from build123d import *

# Parameters (mm, degrees)
SKETCH1_W           = 45
SKETCH1_H           = 250
BOSS_EXTRUDE1_DEPTH = 12
SKETCH2_W           = 5
SKETCH2_H           = 105
CUT_EXTRUDE1_DEPTH  = 12
SKETCH3_R           = 1.75
CUT_EXTRUDE2_DEPTH  = 35
SKETCH5_W           = 25
SKETCH5_H           = 30
SKETCH5_W_2         = 5
BOSS_EXTRUDE2_DEPTH = 12
SKETCH7_R           = 12
SKETCH7_R_2         = 1.25
CUT_EXTRUDE3_DEPTH  = 35
SKETCH8_W           = 18
SKETCH8_H           = 11
CUT_EXTRUDE4_DEPTH  = 12
SKETCH10_R          = 11
CUT_EXTRUDE5_DEPTH  = 7
SKETCH11_W          = 45
SKETCH11_H          = 20
CUT_EXTRUDE6_DEPTH  = 20
FILLET3_R           = 5
SKETCH12_R          = 5
CUT_EXTRUDE7_DEPTH  = 10
SKETCH13_R          = 1.5
CUT_EXTRUDE8_DEPTH  = 12
CUT_EXTRUDE9_DEPTH  = 20
FILLET4_R           = 18
SKETCH15_R          = 5
CUT_EXTRUDE10_DEPTH = 10


with BuildPart() as part:
    # Sketch1 → Boss-Extrude1 (new body)
    with BuildSketch(Plane(origin=(0, 0, 0), x_dir=(1, 0, 0), z_dir=(0, 1, 0))):
        Rectangle(SKETCH1_W, SKETCH1_H)
    extrude(amount=BOSS_EXTRUDE1_DEPTH)

    # Sketch2 → Cut-Extrude1 (cut)
    with BuildSketch(Plane(origin=(0, 12, 0), x_dir=(1, 0, 0), z_dir=(0, 1, 0))):
        with Locations((20, 42.5)):
            Rectangle(SKETCH2_W, SKETCH2_H)
        with Locations((-20, 42.5)):
            Rectangle(SKETCH2_W, SKETCH2_H)
    extrude(amount=-CUT_EXTRUDE1_DEPTH, mode=Mode.SUBTRACT)

    # Sketch3 → Cut-Extrude2 (cut)
    with BuildSketch(Plane(origin=(17.5, 0, 0), x_dir=(0, 0, -1), z_dir=(1, 0, 0))):
        with Locations((15, 6)):
            Circle(SKETCH3_R)
        with Locations((75, 6)):
            Circle(SKETCH3_R)
    extrude(amount=-CUT_EXTRUDE2_DEPTH, mode=Mode.SUBTRACT)

    # Sketch5 → Boss-Extrude2 (add)
    with BuildSketch(Plane(origin=(0, 12, 0), x_dir=(1, 0, 0), z_dir=(0, 1, 0))):
        with Locations((35, 110)):
            Rectangle(SKETCH5_W, SKETCH5_H)
        with Locations((-25, 110)):
            Rectangle(SKETCH5_W_2, SKETCH5_H)
    extrude(amount=-BOSS_EXTRUDE2_DEPTH)

    # Sketch7 → Cut-Extrude3 (cut)
    with BuildSketch(Plane(origin=(0, 12, 0), x_dir=(1, 0, 0), z_dir=(0, 1, 0))):
        with Locations(Location((0, 110, 0), (0, 0, 270))):
            Circle(SKETCH7_R)
        with Locations(Location((21.920310217, 110, 0), (0, 0, 270))):
            Circle(SKETCH7_R_2)
        with Locations(Location((-21.920310217, 110, 0), (0, 0, 270))):
            Circle(SKETCH7_R_2)
        with Locations(Location((0, 88.079689783, 0), (0, 0, 270))):
            Circle(SKETCH7_R_2)
    extrude(amount=-CUT_EXTRUDE3_DEPTH, mode=Mode.SUBTRACT)

    # Sketch8 → Cut-Extrude4 (cut)
    with BuildSketch(Plane(origin=(0, 12, 0), x_dir=(1, 0, 0), z_dir=(0, 1, 0))):
        with Locations((38.5, 119.5)):
            Rectangle(SKETCH8_W, SKETCH8_H)
    extrude(amount=-CUT_EXTRUDE4_DEPTH, mode=Mode.SUBTRACT)

    # Sketch10 → Cut-Extrude5 (cut)
    with BuildSketch(Plane(origin=(0, 12, 0), x_dir=(1, 0, 0), z_dir=(0, 1, 0))):
        with Locations(Location((0, 12.25, 0), (0, 0, 270))):
            Circle(SKETCH10_R)
        with Locations(Location((0, -85.5, 0), (0, 0, 270))):
            Circle(SKETCH10_R)
    extrude(amount=-CUT_EXTRUDE5_DEPTH, mode=Mode.SUBTRACT)

    # Sketch11 → Cut-Extrude6 (cut)
    with BuildSketch(Plane(origin=(0, 12, 0), x_dir=(1, 0, 0), z_dir=(0, 1, 0))):
        with Locations((0, -115)):
            Rectangle(SKETCH11_W, SKETCH11_H)
    extrude(amount=-CUT_EXTRUDE6_DEPTH, mode=Mode.SUBTRACT)

    # Fillet3
    fillet3_edges = [part.edges().sort_by_distance(p)[0] for p in [
        (29.5, 6, -114),
    ]]
    fillet(fillet3_edges, radius=FILLET3_R)

    # Sketch12 → Cut-Extrude7 (cut)
    with BuildSketch(Plane(origin=(0, 5, 0), x_dir=(1, 0, 0), z_dir=(0, 1, 0))):
        with Locations(Location((0, -85.5, 0), (0, 0, 270))):
            Circle(SKETCH12_R)
        with Locations(Location((0, 12.25, 0), (0, 0, 270))):
            Circle(SKETCH12_R)
    extrude(amount=-CUT_EXTRUDE7_DEPTH, mode=Mode.SUBTRACT)

    # Sketch13 → Cut-Extrude8 (cut)
    with BuildSketch(Plane(origin=(0, 12, 0), x_dir=(1, 0, 0), z_dir=(0, 1, 0))):
        with Locations(Location((38, 104.5, 0), (0, 0, 270))):
            Circle(SKETCH13_R)
        with Locations(Location((44, 104.5, 0), (0, 0, 270))):
            Circle(SKETCH13_R)
    extrude(amount=-CUT_EXTRUDE8_DEPTH, mode=Mode.SUBTRACT)

    # Sketch14 → Cut-Extrude9 (cut)
    with BuildSketch(Plane(origin=(0, 12, 0), x_dir=(1, 0, 0), z_dir=(0, 1, 0))):
        Polygon((-22.5, -20), (-22.5, -105), (-17.5, -105), align=None)
        Polygon((17.5, -105), (22.5, -20), (22.5, -105), align=None)
    extrude(amount=-CUT_EXTRUDE9_DEPTH, mode=Mode.SUBTRACT)

    # Fillet4
    fillet4_edges = [part.edges().sort_by_distance(p)[0] for p in [
        (17.5, 6, 105),
        (-17.5, 6, 105),
    ]]
    fillet(fillet4_edges, radius=FILLET4_R)

    # Sketch15 → Cut-Extrude10 (cut)
    with BuildSketch(Plane(origin=(0, 12, 0), x_dir=(1, 0, 0), z_dir=(0, 1, 0))):
        with Locations(Location((0, 67.5, 0), (0, 0, 270))):
            Circle(SKETCH15_R)
    extrude(amount=-CUT_EXTRUDE10_DEPTH, mode=Mode.SUBTRACT)


solid = part.part
Model file for the job. Use its own axes, mm. A direction names the side the tool comes from. Coordinates: 2 decimals unless noted, no trailing zeros. Order: outer loops, then holes, each group sorted by start corner. A loop starts at its lowest first (then second) coordinate and runs counter-clockwise, first axis right, second up. Notation, with made-up numbers: M 29,62 L 70,62 A8 ccw 70,74 Z; hole C 5,85.25 d4. An arc over 180 degrees is marked long. Return JSON: item names as keys, results as strings.
1. Saw through at C-C (z = -21). Give the cut face in (x, y).
Ans:
{"outline": "M -17.5,0 L 17.5,0 L 17.5,12 L 6.67,12 L 6.67,5 L -6.67,5 L -6.67,12 L -17.5,12 Z"}
2. Saw through at D-D (z = -69.5). Give the cut face in (x, y).
Ans:
{"outline": "M -17.5,0 L 17.5,0 L 17.5,12 L 4.58,12 L 4.58,2 L -4.58,2 L -4.58,12 L -17.5,12 Z"}
3. Tool access for faces 4 (the face through (29.5, 6, -122)), 5 (the face through (-17.5, 6, -42)), 6 (the face through (0, 5, -6)), 7 (the face through (32, 6, -95)), 8 (the face through (22.5, 6, 15)): list every direction of +Z, -Z, +X, -X, +Y, -Y with a clear straight run to the whole face (end or side of a thin tool).
Ans:
{"face 4": "-Z, +X, +Y, -Y", "face 5": "-X, +Y, -Y", "face 6": "+Y", "face 7": "+X, +Y, -Y", "face 8": "+Z, +X, +Y, -Y"}
4. Saw through at A-A (x = 14.5). Give the cut face in (y, z), and give its area (3 significant figures).
Ans:
{"outline": "M 0,-125 L 12,-125 L 12,98.35 L 0,98.35 Z; hole C 6,-75 d3.5; hole C 6,-15 d3.5", "area": "2,660 mm^2"}
5. Drill centre lines: probe 1 along X at (y, z) = (8.25, -104.5); probe 2 along X at (y, z) = (8.25, -67.5); probe 3 along X at (y, z) = (10.5, -12.25). Where is each one in solid material? Low to high.
Ans:
{"probe 1": "-27.5 to -10.67, 10.67 to 36.5, 39.5 to 42.5, 45.5 to 47.5", "probe 2": "-17.5 to -5, 5 to 17.5", "probe 3": "-17.5 to -11, 11 to 17.5"}
6. Flat gauge pins, fed straight in: pin 1 (17.5 mm diameter, centred on x = 0, z = 85.5, fed in from +Y); pin 2 (4 mm diameter, centred on x = -5, y = 6.5, fed in from +Z); pin 3 (5 mm diameter, centred on y = 6, z = 17, fed in from +X). Where does each tip first touch, or does it go through?
Ans:
{"pin 1": "y = 5", "pin 2": "z = 104.83", "pin 3": "x = 22.5"}
7. Saw through at B-B (z = 85.5). Give the cut face in (x, y), and give its area (3 significant figures).
Ans:
{"outline": "M -18.65,0 L -5,0 L -5,5 L -11,5 L -11,12 L -18.65,12 Z; M 5,0 L 18.65,0 L 18.65,12 L 11,12 L 11,5 L 5,5 Z", "area": "244 mm^2"}
8. Pull direction X, two halves, no side cores. Call faces 1 (the face through (-20, 6, 10)), 2 (the face through (-1.915, 7.07, -62.881)), 3 (the face through (47.5, 6, -104)): +X half, -X half, draft (parallel to the pull), parting line (faces both ways), or undercut.
Ans:
{"face 1": "draft", "face 2": "undercut", "face 3": "+X half"}
